```python
from build123d import *

# Parameters (mm, degrees)
BOSS_EXTRUDE1_DEPTH      = 22.46
BOSS_EXTRUDE1_DEPTH_BACK = 3.81
SKETCH1_W                = 10
SKETCH1_H                = 25.4
SKETCH4_R                = 1.5
CUT_EXTRUDE1_DEPTH       = 6.35
SKETCH5_R                = 1.5
CUT_EXTRUDE2_DEPTH       = 250
BOSS_EXTRUDE2_START      = -6.35
BOSS_EXTRUDE2_OUTLINE_R  = 1.5
BOSS_EXTRUDE2_DEPTH      = 6.35
FILLET1_R                = 5.08


# Read off the part's stored shape, not the designer's step: Boss-Extrude2
with BuildPart() as part:
    # Sketch1 → Boss-Extrude1 (new, two sides: drawn at the far end of the back side and taken through both)
    with BuildSketch(Plane(origin=(0, 0, 0), x_dir=(1, 0, 0), z_dir=(0, 1, 0)).offset(-BOSS_EXTRUDE1_DEPTH_BACK)):
        with Locations((5, 12.7)):
            Rectangle(SKETCH1_W, SKETCH1_H)
    extrude(amount=BOSS_EXTRUDE1_DEPTH + BOSS_EXTRUDE1_DEPTH_BACK)

    # Sketch4 → Cut-Extrude1 (cut)
    with BuildSketch(Plane(origin=(10, 0, 0), x_dir=(0, 0, -1), z_dir=(1, 0, 0))):
        with Locations((19.771067812, 1.818932188)):
            Circle(SKETCH4_R)
        with Locations((5.628932188, 1.818932188)):
            Circle(SKETCH4_R)
        with Locations((5.628932188, 15.961067812)):
            Circle(SKETCH4_R)
        with Locations((19.771067812, 15.961067812)):
            Circle(SKETCH4_R)
    extrude(amount=-CUT_EXTRUDE1_DEPTH, mode=Mode.SUBTRACT)

    # Sketch5 → Cut-Extrude2 (cut)
    with BuildSketch(Plane(origin=(10, 0, 0), x_dir=(0, 0, -1), z_dir=(1, 0, 0))):
        with Locations((13.361067812, 17.551067934)):
            Circle(SKETCH5_R)
        with Locations((13.361067812, 0.231067934)):
            Circle(SKETCH5_R)
        with Locations(Location((3.361067812, 0.231067934, 0), (0, 0, 12.341353826))):
            Circle(SKETCH5_R)
        with Locations(Location((3.361067812, 17.551067934, 0), (0, 0, 347.561610905))):
            Circle(SKETCH5_R)
    extrude(amount=-CUT_EXTRUDE2_DEPTH, mode=Mode.SUBTRACT)

    # Boss-Extrude2 outline → Boss-Extrude2 (add)
    with BuildSketch(Plane(origin=(10, 0, 0), x_dir=(0, 0, -1), z_dir=(1, 0, 0)).offset(BOSS_EXTRUDE2_START)):
        with BuildLine():
            ThreePointArc((4.163594844, 1.498328903), (2.132311367, -0.629256191), (4.826405157, 0.551671219))
            ThreePointArc((4.826405157, 0.551671219), (4.400175743, 0.958608063), (4.163594844, 1.498328903))
        make_face()
        with BuildLine():
            ThreePointArc((4.825860086, 17.227983436), (2.132855084, 18.412168099), (4.164139914, 16.28415231))
            ThreePointArc((4.164139914, 16.28415231), (4.400719459, 16.822167976), (4.825860086, 17.227983436))
        make_face()
        with Locations((13.361067812, 0.231067934)):
            Circle(BOSS_EXTRUDE2_OUTLINE_R)
        with Locations((13.361067812, 17.551067934)):
            Circle(BOSS_EXTRUDE2_OUTLINE_R)
    extrude(amount=BOSS_EXTRUDE2_DEPTH)

    # Fillet1
    fillet1_edges = [part.edges().sort_by_distance(p)[0] for p in [
        (5, 22.46, 0),
        (5, 22.46, -25.4),
        (5, -3.81, -25.4),
        (5, -3.81, 0),
    ]]
    fillet(fillet1_edges, radius=FILLET1_R)


solid = part.part
```
Can you work these out from the model? Positions are in its coordinate system, mm. A direction names the side the tool comes from. Give positions to 0.01 mm unless a question says otherwise; leave off trailing zeros. Order: outer loops, then holes, each group sorted by start corner. A loop starts at its lowest first (then second) coordinate and runs counter-clockwise, first axis right, second up. Notation, with made-up numbers: M 46.5,0.5 L 69.5,0.5 A17 cw 69.5,27.5 Z; hole C 49,75 d2. An arc over 180 degrees is marked long. Write item = value, one per line. Start each with the question number.
Q1. We'd pull the mould along Z, two halves only. Please class faces 1 (the cylindrical face through (5.07, 20.932, -1.449)), 2 (the flat face through (5, 9, -25.4)), 3 (the flat face through (0, 9, -13)), 4 (the flat face through (3.65, 18, -13)): pulls with the +Z half, pulls with the -Z half, needs draft (parallel to the pull), parting line crosses it, or undercut.
Q2. Suppose I cut it at A-A (x = 8). Write out the boundary of the cut face in (y, z).
Q3. Will these pins go through, and if not, where does the flat tip stop? pin 1 Ø0.9 at (y, z) = (1, -14) entering from -X; pin 2 Ø0.9 at (y, z) = (1.5, -5) entering from +X.
Q4. Suppose I cut it at C-C (y = -0.25). Write out the boundary of the cut face in (x, z).
Q5. Suppose I cut it at B-B (z = -14.5). Write out the boundary of the cut face in (x, y).
Q6. For faces 5 (the flat face through (3.65, 0, -3)), 6 (the flat face through (3.65, 16, -6)), 7 (the flat face through (10, 10, -13)), which set-ups out of +Z, -Z, +X, -X, +Y, -Y let a thin tool reach every point of the face, with its end or its side?
Q7. I need wall thicknesses on probe 1 along Y at (x, z) = (9, -18.75); probe 2 along Z at (x, y) = (7.5, 2.25); probe 3 along X at (y, z) = (18.25, -13). Which ranges of each line are inside material? Lowest first, please. Write a range as [from, to].
Q8. Suppose I cut it at D-D (z = -22.5). Write out the boundary of the cut face in (x, y), plus the area to 3 significant figures.
Check result:
q1.face_1 = pulls with the +Z half
q1.face_2 = pulls with the -Z half
q1.face_3 = needs draft
q1.face_4 = undercut
q2.outline = M -3.81,-20.32 A5.08 ccw 1.27,-25.4 L 17.38,-25.4 A5.08 ccw 22.46,-20.32 L 22.46,-5.08 A5.08 ccw 17.38,0 L 1.27,0 A5.08 ccw -3.81,-5.08 Z; hole C 1.82,-19.77 d3; hole C 1.82,-5.63 d3; hole C 15.96,-19.77 d3; hole C 15.96,-5.63 d3
q3.pin_1 = 3.65
q3.pin_2 = 3.65
q4.outline = M 0,-25.17 L 10,-25.17 L 10,-0.23 L 0,-0.23 L 0,-1.94 L 3.65,-1.94 L 3.65,-4.78 L 0,-4.78 L 0,-11.94 L 3.65,-11.94 L 3.65,-14.78 L 0,-14.78 Z
q5.outline = M 0,-3.81 L 10,-3.81 L 10,22.46 L 0,22.46 L 0,18.53 L 3.65,18.53 L 3.65,16.57 L 0,16.57 L 0,1.21 L 3.65,1.21 L 3.65,-0.75 L 0,-0.75 Z
q6.face_5 = -X
q6.face_6 = +X
q6.face_7 = +Z, -Z, +X, +Y, -Y
q7.probe_1 = [-3.81, 0.72], [2.92, 14.86], [17.06, 22.46]
q7.probe_2 = [-25.4, -21.21], [-18.33, -7.07], [-4.19, 0]
q7.probe_3 = [3.65, 10]
q8.outline = M 0,-3.32 L 10,-3.32 L 10,21.97 L 0,21.97 Z
q8.area = 253 mm2
